Autodesk Inventor part; units mm, degrees
ref_plane "YZ Plane" through (0, 0, 0) normal (1, 0, 0) x (0, 1, 0)
ref_plane "XZ Plane" through (0, 0, 0) normal (0, 1, 0) x (-1, 0, 0)
ref_plane "XY Plane" through (0, 0, 0) normal (0, 0, 1) x (1, 0, 0)
sketch "Sketch1" plane through (0, 0, 0) normal (0, 0, 1) x (1, 0, 0)
  line L0 (0, 0) -> (60, 0)
  line L1 (60, 0) -> (60, 10)
  line L2 (60, 10) -> (0, 10)
  line L3 (0, 10) -> (0, 0)
  line L4 (0, 0) -> (0, 5) construction
  line L5 (0, 5) -> (5, 5) construction
  circle A0 centre (5, 5) radius 1.5
  circle A1 centre (55, 5) radius 1.5
  dimension "d0" = 60
  dimension "d1" = 10
  dimension "d2" = 5
  dimension "d3" = 5
  dimension "d4" = 3
  dimension "d5" = 3
  dimension "d6" = 5
  dimension "d7" = 5
extrude "Extrusion1" add sketch "Sketch1" along normal blind 60
sketch "Sketch2" plane through (0, 10, 0) normal (0, 1, 0) x (1, 0, 0)
  circle A0 centre (30, -30.8633) radius 17.5
  line L0 (0, 0) -> (0, -60)
  line L1 (60, 0) -> (0, 0)
  dimension "d10" = 35
  dimension "d12" = 30
  dimension "d13" = 30.8633
extrude "Extrusion2" cut sketch "Sketch2" against normal blind 10
fillet "Fillet1" radius 5 6 edges at (0, 10, 30) (60, 10, 30) (60, 0, 30) (0, 0, 30) (12.5, 0, 30.8633) (12.5, 10, 30.8633)
properties part number "60x10SlimGrommet"
The listing builds one solid part. Answer for the finished solid, in the listing's coordinates (mm). Give positions to 0.01 mm unless a question says otherwise; leave off trailing zeros. Order: outer loops, then holes, each group sorted by start corner. A loop starts at its lowest first (then second) coordinate and runs counter-clockwise, first axis right, second up. Notation, with made-up numbers: (-11, 17.5) -> (8, 17.5) arc R10 cw to (8, 22.5) -> close; hole circle Ø5 at (27.25, 20.5). An arc over 180 degrees is marked (long way). Write each question's results on one line, items separated by ' | '.
Q1. Each of these flat-tipped pins is pushed along its axis until it touches: P1, Ø1.5, axis at x = 44.5, z = 6, coming from the -Y side; P2, Ø1, axis at x = 45.5, z = 24.5, coming from the -Y side; P3, Ø3, axis at y = 8, z = 50, coming from the -X side; P4, Ø4, axis at y = 2, z = 16, coming from the -X side. Where does it stop, or does it pass through?
Checked values:
P1: stops at y = 0 | P2: passes through | P3: stops at x = 0.23 | P4: stops at x = 0.1
Q2. The part is cut by section B-B, the plane y = 5.75. Give the vertices of the cut face in (x, z), and give its area (3 significant figures).
Checked values:
outline: (0.06, 0) -> (3.7, 0) -> (3.7, 60) -> (0.06, 60) -> close; (6.3, 0) -> (53.7, 0) -> (53.7, 60) -> (6.3, 60) -> close; (56.3, 0) -> (59.94, 0) -> (59.94, 60) -> (56.3, 60) -> close; hole circle Ø35.11 at (30, 30.86) | area: 2,310 mm^2
Q3. Straight lines are drawn through the part: probe 1 along Y at (x, z) = (55, 30); probe 2 along X at (y, z) = (4, 42.5); probe 3 along Z at (x, y) = (30, 5.05). For each, find the intervals that lie inside material, in ascending order. Write a range as from..to.
Checked values:
probe 1: y = 0..3.5, 6.5..10 | probe 2: x = 0.1..3.88, 6.12..16.79, 43.21..53.88, 56.12..59.9 | probe 3: z = 0..13.36, 48.36..60
Q4. The part is cut by section C-C, the plane y = 2.75. Give the vertices of the cut face in (x, z), and give its area (3 significant figures).
Checked values:
outline: (0.53, 0) -> (59.47, 0) -> (59.47, 60) -> (0.53, 60) -> close; hole circle Ø36.07 at (30, 30.86) | area: 2,510 mm^2
Q5. The part is cut by section A-A, the plane z = 7. State how many separate pieces and enclosed holes the cut face has, and give its area (3 significant figures).
Checked values:
separate pieces: 1 | enclosed holes: 2 | area: 564 mm^2
